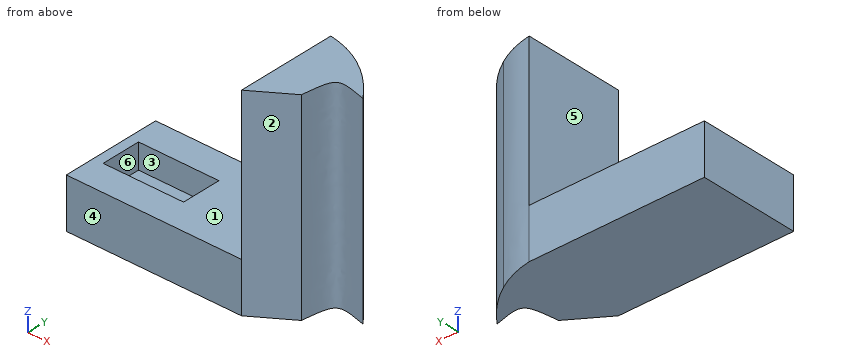
```python
from build123d import *

# Parameters (mm, degrees)
F0_W      = 101.6
F0_H      = 50.8
F1_DEPTH  = 25.4
F3_DEPTH  = 12.7
F4_W      = 12.7
F4_H      = 50.8
F5_DEPTH  = 76.2
F6_DEPTH  = 25.4
F8_DEPTH  = 228.6
F10_DEPTH = 228.6
F12_DEPTH = 228.6


with BuildPart() as f1:
    # F0 (on Top) → F1 (new body)
    with BuildSketch(Plane.XY):
        Rectangle(F0_W, F0_H)
    extrude(amount=F1_DEPTH)

    # F2 (on face) → F3 (cut)
    with BuildSketch(Plane.XY.offset(25.4)):
        with BuildLine():
            Line((-22.7059231637, 2.6940768363), (-25.4, 0))
            Line((-25.4, 0), (-22.7059231637, -2.6940768363))
            ThreePointArc((-22.7059231637, -2.6940768363), (-21.8800189811, -1.4580238773), (-21.59, 0))
            ThreePointArc((-21.59, 0), (-21.8800189811, 1.4580238773), (-22.7059231637, 2.6940768363))
        make_face()
        with BuildLine():
            ThreePointArc((-22.7059231637, 2.6940768363), (-25.4, 3.81), (-28.0940768363, 2.6940768363))
            Line((-28.0940768363, 2.6940768363), (-25.4, 0))
            Line((-25.4, 0), (-22.7059231637, 2.6940768363))
        make_face()
        with BuildLine():
            Line((-25.4, 0), (-28.0940768363, 2.6940768363))
            ThreePointArc((-28.0940768363, 2.6940768363), (-29.21, 0), (-28.0940768363, -2.6940768363))
            Line((-28.0940768363, -2.6940768363), (-25.4, 0))
        make_face()
        with BuildLine():
            Line((-22.7059231637, -2.6940768363), (-25.4, 0))
            Line((-25.4, 0), (-28.0940768363, -2.6940768363))
            ThreePointArc((-28.0940768363, -2.6940768363), (-25.4, -3.81), (-22.7059231637, -2.6940768363))
        make_face()
        with BuildLine():
            Line((-5.0000027, 10.05000022), (-14.7721255415, 10.05000022))
            ThreePointArc((-14.7721255415, 10.05000022), (-11.8093784333, 5.4082552971), (-10.772825976, 0))
            ThreePointArc((-10.772825976, 0), (-11.8093784333, -5.4082552971), (-14.7721255415, -10.05000022))
            Line((-14.7721255415, -10.05000022), (-5.0000027, -10.05000022))
            Line((-5.0000027, -10.05000022), (-5.0000027, 10.05000022))
        make_face()
        with BuildLine():
            Line((-15.34999978, 10.05000022), (-35.45000022, 10.05000022))
            Line((-35.45000022, 10.05000022), (-28.0940768363, 2.6940768363))
            ThreePointArc((-28.0940768363, 2.6940768363), (-25.4, 3.81), (-22.7059231637, 2.6940768363))
            Line((-22.7059231637, 2.6940768363), (-15.34999978, 10.05000022))
        make_face()
        with BuildLine():
            Line((-28.0940768363, -2.6940768363), (-35.45000022, -10.05000022))
            Line((-35.45000022, -10.05000022), (-15.34999978, -10.05000022))
            Line((-15.34999978, -10.05000022), (-22.7059231637, -2.6940768363))
            ThreePointArc((-22.7059231637, -2.6940768363), (-25.4, -3.81), (-28.0940768363, -2.6940768363))
        make_face()
        with BuildLine():
            ThreePointArc((-36.0278744585, -10.05000022), (-40.027174024, 0), (-36.0278744585, 10.05000022))
            Line((-36.0278744585, 10.05000022), (-45.7999973, 10.05000022))
            Line((-45.7999973, 10.05000022), (-45.7999973, -10.05000022))
            Line((-45.7999973, -10.05000022), (-36.0278744585, -10.05000022))
        make_face()
        with BuildLine():
            Line((-14.7721255415, 10.05000022), (-15.34999978, 10.05000022))
            Line((-15.34999978, 10.05000022), (-22.7059231637, 2.6940768363))
            ThreePointArc((-22.7059231637, 2.6940768363), (-21.8800189811, 1.4580238773), (-21.59, 0))
            ThreePointArc((-21.59, 0), (-21.8800189811, -1.4580238773), (-22.7059231637, -2.6940768363))
            Line((-22.7059231637, -2.6940768363), (-15.34999978, -10.05000022))
            Line((-15.34999978, -10.05000022), (-14.7721255415, -10.05000022))
            ThreePointArc((-14.7721255415, -10.05000022), (-11.8093784333, -5.4082552971), (-10.772825976, 0))
            ThreePointArc((-10.772825976, 0), (-11.8093784333, 5.4082552971), (-14.7721255415, 10.05000022))
        make_face()
        with BuildLine():
            Line((-28.0940768363, 2.6940768363), (-35.45000022, 10.05000022))
            Line((-35.45000022, 10.05000022), (-36.0278744585, 10.05000022))
            ThreePointArc((-36.0278744585, 10.05000022), (-40.027174024, 0), (-36.0278744585, -10.05000022))
            Line((-36.0278744585, -10.05000022), (-35.45000022, -10.05000022))
            Line((-35.45000022, -10.05000022), (-28.0940768363, -2.6940768363))
            ThreePointArc((-28.0940768363, -2.6940768363), (-29.21, 0), (-28.0940768363, 2.6940768363))
        make_face()
    extrude(amount=-F3_DEPTH, mode=Mode.SUBTRACT)

    # F4 (on face) → F5 (join)
    with BuildSketch(Plane.XY.offset(25.4)):
        with Locations((44.45, 0)):
            Rectangle(F4_W, F4_H)
    extrude(amount=F5_DEPTH)

    # F6 (add): a face of the model
    f6_faces = [f1.faces().sort_by_distance(p)[0] for p in [
        (50.8, 0, 50.8),
    ]]
    extrude(f6_faces, amount=F6_DEPTH)

    # F7 (on face) → F8 (cut)
    with BuildSketch(Plane.XY.offset(101.6)):
        with BuildLine():
            Line((57.15, 25.4), (38.1, 25.4))
            add(Edge.make_bspline(
                [(38.1, 25.4), (45.2961309058, 24.4295362641), (51.659373316, 21.8816089912), (57.15, 18.5792745817)],
                knots=[0, 0, 0, 0, 8.5975400143, 8.5975400143, 8.5975400143, 8.5975400143], degree=3))
            Line((57.15, 18.5792745817), (57.15, 25.4))
        make_face()
        with BuildLine():
            Line((76.2, 25.4), (57.15, 25.4))
            Line((57.15, 25.4), (57.15, 18.5792745817))
            add(Edge.make_bspline(
                [(57.15, 18.5792745817), (65.6305263938, 13.4786666307), (72.0293207641, 6.57832777), (76.2, 0.9109777383)],
                knots=[8.5975400143, 8.5975400143, 8.5975400143, 8.5975400143, 21.8768374808, 21.8768374808, 21.8768374808, 21.8768374808], degree=3))
            Line((76.2, 0.9109777383), (76.2, 25.4))
        make_face()
    extrude(amount=-F8_DEPTH, mode=Mode.SUBTRACT)

    # F9 (on face) → F10 (cut)
    with BuildSketch(Plane.XY.offset(101.6)):
        Polygon((38.1, -25.4), (57.15, -25.4), (57.15, -12.7636595487), align=None)
    extrude(amount=-F10_DEPTH, mode=Mode.SUBTRACT)

    # F11 (on face) → F12 (cut)
    with BuildSketch(Plane.XY.offset(101.6)):
        with BuildLine():
            add(Edge.make_bspline(
                [(57.15, -12.7636595487), (59.5569387078, 5.385174416), (59.5569387078, 5.385174416), (76.2, 0.9109777382)],
                knots=[0, 0, 0, 0, 23.4499084205, 23.4499084205, 23.4499084205, 23.4499084205], degree=3))
            Line((57.15, -12.7636595487), (57.15, -25.4))
            Line((57.15, -25.4), (76.2, -25.4))
            Line((76.2, -25.4), (76.2, 0.9109777383))
        make_face()
    extrude(amount=-F12_DEPTH, mode=Mode.SUBTRACT)


solid = f1.part
```
Geometry check sheet. Reference: the model listing, model coordinates, mm. Face numbers are marked on the shaded views. A direction names the side the tool comes from. Coordinates: 2 decimals unless noted, no trailing zeros. Loops run counter-clockwise (first coordinate to the right, second up) from the corner with the lowest first, then second, coordinate; pieces in that order, holes last.
Item 1: Sectioned sample at C-C, the plane x = 15.5. Record the boundary of the cut face in (y, z), then the cut area to 3 significant figures.
Item 2: Sectioned sample at B-B, the plane y = -19.5. Record the boundary of the cut face in (x, z).
Item 3: Access from +Z, -Z, +X, -X, +Y, -Y to the whole of each face (thin tool, end or side, straight path). Record for the marked faces 4, 5 and 6.
Item 4: Release check for a two-part mould opening along Y. For the marked faces 1, 2 and 3 record: released by +Y, released by -Y, zero draft, split by the parting line, or undercut.
Item 5: Sectioned sample at A-A, the plane x = -14. Record the boundary of the cut face in (y, z), then the cut area to 3 significant figures.
Item 6: Thickness scan on line 1 (Z direction, x = -2, y = 1); line 2 (Z direction, x = -35, y = 2.5); line 3 (X direction, y = -16.5, z = 84.5). Record the ranges inside material, lowest first.
Item 7: Go/stop test with flat-tipped pins: pin 1 Ø2 at (x, y) = (13, 9.5) entering from +Z; pin 2 Ø12 at (x, z) = (63, 91) entering from +Y; pin 3 Ø10 at (x, y) = (-15.5, 4) entering from +Z. Record where each tip stops, or that it passes through.
Check result:
1. outline: (-25.4, 0) - (25.4, 0) - (25.4, 25.4) - (-25.4, 25.4) - close
1. area: 1,290 mm2
2. outline: (-50.8, 0) - (46.99, 0) - (46.99, 101.6) - (38.1, 101.6) - (38.1, 25.4) - (-50.8, 25.4) - close
3. face 4: +Z, -Z, +X, -X, -Y
3. face 5: +Z, -X, +Y, -Y
3. face 6: +Z
4. face 1: zero draft
4. face 2: released by -Y
4. face 3: undercut
5. outline: (-25.4, 0) - (25.4, 0) - (25.4, 25.4) - (10.05, 25.4) - (10.05, 12.7) - (-10.05, 12.7) - (-10.05, 25.4) - (-25.4, 25.4) - close
5. area: 1,040 mm2
6. line 1: z = 0 to 25.4
6. line 2: z = 0 to 12.7
6. line 3: x = 38.1 to 51.52
7. pin 1: stops at z = 25.4
7. pin 2: stops at y = 18.67
7. pin 3: stops at z = 12.7
